Read the model definition and answer for the solid it produces. Units are mm, in the model's axes. A direction names the side the tool comes from. Coordinates: 2 decimals unless noted, no trailing zeros. Write each loop counter-clockwise with the first axis right and the second up, starting at its lowest first coordinate (ties: lowest second). Pieces come first, ordered by that corner, then holes.
1) The part is cut by section C-C (x = -24.5). Determine the outline of the cut face in (y, z), then the cut area to 3 significant figures.
2) Find the intervals of material crossed by line 1 (X direction, y = 0.9, z = 19.5); line 2 (X direction, y = 1, z = -19); line 3 (Y direction, x = -22, z = 16.5), in increasing order.
3) The part is cut by section B-B (z = 13). Determine the outline of the cut face in (x, y), then the cut area to 3 significant figures.
4) The part is cut by section A-A (x = -17.5). Determine the outline of the cut face in (y, z).
5) The part is cut by section D-D (z = 20). Determine the outline of the cut face in (x, y), then the cut area to 3 significant figures.
6) Determine the mould class of faces 4 (the face through (-25.5, 1, 0)), 5 (the face through (8.6, 4.9, 0.3)), 6 (the face through (-24.621, 0.986, -22.247)), 7 (the face through (-30, 1, 0)) for opening direction X: +X half, -X half, draft (parallel to the pull), parting line (faces both ways), or undercut.
7) Each of these flat-tipped pins is pushed along its axis until it touches: pin 1 Ø2 at (y, z) = (25, 9.5) entering from +X; pin 2 Ø0.6 at (y, z) = (0.5, -3) entering from +X; pin 3 Ø2 at (y, z) = (37.5, -18.5) entering from +X. Where does it stop, or does it pass through?
8) Which of the six approach directions +Z, -Z, +X, -X, +Y, -Y give full straight-line access (tool end or side, diameter ignored) to faces 1 (the face through (-10.379, 0.986, 22.247)), 2 (the face through (-8, 2, 0)), 3 (the face through (-12.19, 49.15, 0.27))?
from build123d import *

# Parameters (mm, degrees)
SM_BASE_FLANGE_1_DEPTH = 24
SKETCH_3_R             = 2.75
CUT_EXTRUDE_1_DEPTH    = 2
SKETCH_4_R             = 11.5
CUT_EXTRUDE_2_DEPTH    = 2
FILLET_1_R             = 5
CUT_EXTRUDE_3_DEPTH    = 2


# Sheet-metal steps are written as plain solids
with BuildPart() as part:
    # Sketch 1 → 基体-法兰1 (new, symmetric)
    with BuildSketch(Plane.XY):
        with BuildLine():
            Line((-30, 0), (0, 0))
            ThreePointArc((0, 0), (8.660254038, 5), (8.660254038, 15))
            Line((8.660254038, 15), (-11.339745962, 49.641016151))
            Line((-11.339745962, 49.641016151), (-13.07179677, 48.641016151))
            Line((-13.07179677, 48.641016151), (6.92820323, 14))
            ThreePointArc((6.92820323, 14), (6.92820323, 6), (0, 2))
            Line((0, 2), (-30, 2))
            Line((-30, 2), (-30, 0))
        make_face()
    extrude(amount=SM_BASE_FLANGE_1_DEPTH, both=True)

    # 草图3 → 切除-拉伸1 (cut)
    with BuildSketch(Plane.XZ):
        with Locations(Location((-24.5, 19.5, 0), (0, 0, 270))):
            Circle(SKETCH_3_R)
        with Locations(Location((-10.5, 19.5, 0), (0, 0, 270))):
            Circle(SKETCH_3_R)
        with Locations(Location((-10.5, -19.5, 0), (0, 0, 90))):
            Circle(SKETCH_3_R)
        with Locations(Location((-24.5, -19.5, 0), (0, 0, 90))):
            Circle(SKETCH_3_R)
    extrude(amount=-CUT_EXTRUDE_1_DEPTH, mode=Mode.SUBTRACT)

    # 草图4 → 切除-拉伸2 (cut)
    with BuildSketch(Plane(origin=(12.990381057, 7.5, 0), x_dir=(0, 0, -1), z_dir=(0.8660254037844363, 0.5000000000000041, 0))):
        with Locations(Location((0, 33.660254038, 0), (0, 0, 90))):
            Circle(SKETCH_4_R)
    extrude(amount=-CUT_EXTRUDE_2_DEPTH, mode=Mode.SUBTRACT)

    # 圆角1
    fillet_1_edges = [part.edges().sort_by_distance(p)[0] for p in [
        (-12.205771366, 49.141016151, 24),
        (-12.205771366, 49.141016151, -24),
    ]]
    fillet(fillet_1_edges, radius=FILLET_1_R)

    # 草图5 → 切除-拉伸3 (cut)
    with BuildSketch(Plane.XZ):
        with BuildLine():
            Line((-9.5, 7.5), (-9.5, -7.5))
            ThreePointArc((-9.5, -7.5), (-17.5, -15.5), (-25.5, -7.5))
            Line((-25.5, -7.5), (-25.5, 7.5))
            ThreePointArc((-25.5, 7.5), (-17.5, 15.5), (-9.5, 7.5))
        make_face()
    extrude(amount=-CUT_EXTRUDE_3_DEPTH, mode=Mode.SUBTRACT)


solid = part.part
Reported:
1. outline: (0, -24) - (2, -24) - (2, -22.25) - (0, -22.25) - close; (0, -16.75) - (2, -16.75) - (2, -11.37) - (0, -11.37) - close; (0, 11.37) - (2, 11.37) - (2, 16.75) - (0, 16.75) - close; (0, 22.25) - (2, 22.25) - (2, 24) - (0, 24) - close
1. area: 28.5 mm2
2. line 1: x = -30 to -27.25, -21.75 to -13.25, -7.75 to 4.15
2. line 2: x = -30 to -27.2, -21.8 to -13.2, -7.8 to 4.36
2. line 3: y = 0 to 2
3. outline: (-30, 0) - (-23.31, 0) - (-23.31, 2) - (-30, 2) - close; (-13.07, 48.64) - (6.93, 14) arc R8 cw to (0, 2) - (-11.69, 2) - (-11.69, 0) - (0, 0) arc R10 ccw to (8.66, 15) - (-11.34, 49.64) - close
3. area: 154 mm2
4. outline: (0, -24) - (2, -24) - (2, -15.5) - (0, -15.5) - close; (0, 15.5) - (2, 15.5) - (2, 24) - (0, 24) - close
5. outline: (-30, 0) - (-27.2, 0) - (-27.2, 2) - (-30, 2) - close; (-21.8, 0) - (-13.2, 0) - (-13.2, 2) - (-21.8, 2) - close; (-13.02, 48.55) - (6.93, 14) arc R8 cw to (0, 2) - (-7.8, 2) - (-7.8, 0) - (0, 0) arc R10 ccw to (8.66, 15) - (-11.29, 49.55) - close
5. area: 156 mm2
6. face 4: undercut
6. face 5: +X half
6. face 6: undercut
6. face 7: -X half
7. pin 1: stops at x = 3.46
7. pin 2: stops at x = 3.92
7. pin 3: stops at x = -3.75
8. face 1: -Y
8. face 2: +Z, -Z, -X
8. face 3: +Z, -Z, -X, +Y
